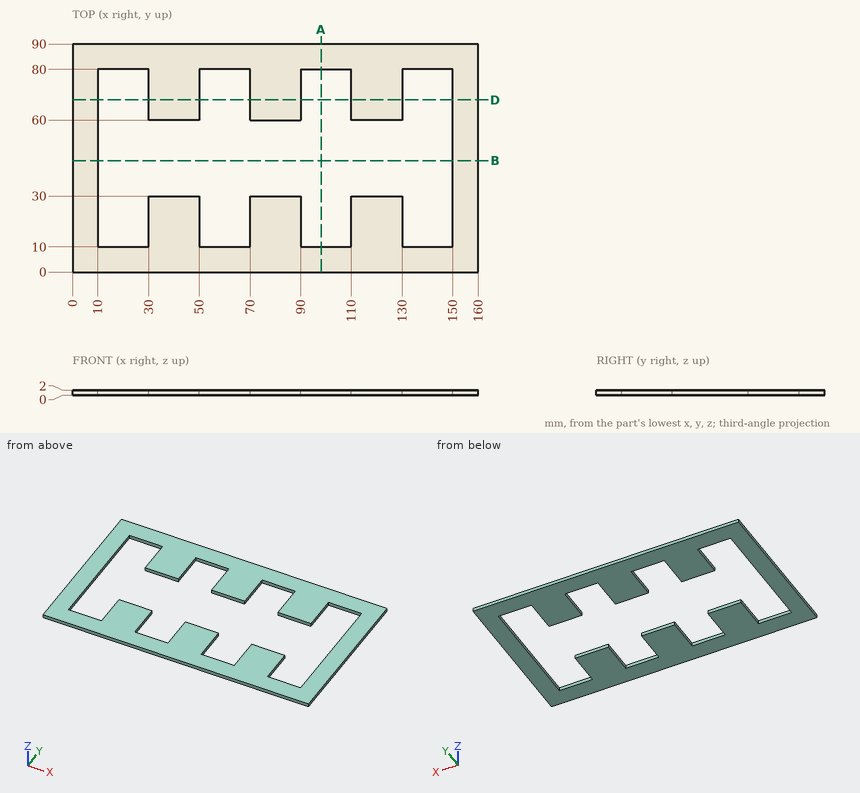
Study the drawing (mm; zero at the part's minimum x, y, z) and answer. Round coordinates to 2 decimals unless told otherwise and drop trailing zeros. Order: outer loops, then holes, each group sorted by start corner. A loop starts at its lowest first (then second) coordinate and runs counter-clockwise, first axis right, second up. Notation, with made-up numbers: (28, -22) -> (66, -22) arc R28 ccw to (66, 15) -> close; hole circle Ø5 at (75, 29.5). An arc over 180 degrees is marked (long way). Answer as CSV lines item,"result". Start each with the question number.
(1) The part is cut by section B-B (y = 44). Determine the outline of the cut face in (x, z).
(2) The part is cut by section D-D (y = 68). Determine the outline of the cut face in (x, z).
(3) Find the intervals of material crossed by probe 1 along X at (y, z) = (16.5, 0.35); probe 2 along X at (y, z) = (31, 1.5); probe 3 along Y at (x, z) = (73.5, 0.25), in increasing order. Write a range as from..to.
(4) The part is cut by section A-A (x = 98). Determine the outline of the cut face in (y, z).
Evaluation:
1,outline,"(0, 0) -> (10, 0) -> (10, 2) -> (0, 2) -> close; (150, 0) -> (160, 0) -> (160, 2) -> (150, 2) -> close"
2,outline,"(0, 0) -> (10, 0) -> (10, 2) -> (0, 2) -> close; (30, 0) -> (50, 0) -> (50, 2) -> (30, 2) -> close; (70, 0) -> (90, 0) -> (90, 2) -> (70, 2) -> close; (110, 0) -> (130, 0) -> (130, 2) -> (110, 2) -> close; (150, 0) -> (160, 0) -> (160, 2) -> (150, 2) -> close"
3,probe 1,"0..10, 30..50, 70..90, 110..130, 150..160"
3,probe 2,"0..10, 150..160"
3,probe 3,"0..30, 60..90"
4,outline,"(0, 0) -> (10, 0) -> (10, 2) -> (0, 2) -> close; (80, 0) -> (90, 0) -> (90, 2) -> (80, 2) -> close"
